from build123d import *

# Parameters (mm, degrees)
BOSS_EXTRUDE1_DEPTH     = 4.4
BOSS_EXTRUDE2_DEPTH     = 1.5
SKETCH3_W               = 42.21
SKETCH3_H               = 37.765
SKETCH3_W_2             = 5.0500889
SKETCH3_H_2             = 9.1998476
SKETCH3_W_3             = 9.1998476
SKETCH3_H_3             = 5.0500889
SKETCH3_W_4             = 12.70002032
SKETCH3_H_4             = 2.54
BOSS_EXTRUDE3_DEPTH     = 1.5
BOSS_EXTRUDE4_START     = -4.4
BOSS_EXTRUDE4_DEPTH     = 4.4
SKETCH4_R               = 0.85
CUT_EXTRUDE1_DEPTH      = 32.45281913
MIRROR2_START           = -4.4
MIRROR2_COPY_1_DEPTH    = 4.4
MIRROR2_COPY_2_SKETCH_R = 0.85
MIRROR2_COPY_2_DEPTH    = 32.45281913
FILLET1_R               = 0.5
SKETCH7_W               = 10
SKETCH7_H               = 1
CUT_EXTRUDE2_DEPTH      = 3
SKETCH8_W               = 1
SKETCH8_H               = 10
CUT_EXTRUDE3_DEPTH      = 3


with BuildPart() as part:
    # Sketch1 → Boss-Extrude1 (new body)
    with BuildSketch(Plane.XY):
        with BuildLine():
            Line((-19.431, 20.8825), (19.431, 20.8825))
            ThreePointArc((19.431, 20.8825), (22.028910314, 19.806410314), (23.105, 17.2085))
            Line((23.105, 17.2085), (23.105, -17.2085))
            ThreePointArc((23.105, -17.2085), (22.028910314, -19.806410314), (19.431, -20.8825))
            Line((19.431, -20.8825), (-19.431, -20.8825))
            ThreePointArc((-19.431, -20.8825), (-22.028910314, -19.806410314), (-23.105, -17.2085))
            Line((-23.105, -17.2085), (-23.105, 17.2085))
            ThreePointArc((-23.105, 17.2085), (-22.028910314, 19.806410314), (-19.431, 20.8825))
        make_face()
        with BuildLine():
            Line((-19.431, -18.8825), (19.431, -18.8825))
            ThreePointArc((19.431, -18.8825), (20.614696752, -18.392196752), (21.105, -17.2085))
            Line((21.105, -17.2085), (21.105, 17.2085))
            ThreePointArc((21.105, 17.2085), (20.614696752, 18.392196752), (19.431, 18.8825))
            Line((19.431, 18.8825), (-19.431, 18.8825))
            ThreePointArc((-19.431, 18.8825), (-20.614696752, 18.392196752), (-21.105, 17.2085))
            Line((-21.105, 17.2085), (-21.105, -17.2085))
            ThreePointArc((-21.105, -17.2085), (-20.614696752, -18.392196752), (-19.431, -18.8825))
        make_face(mode=Mode.SUBTRACT)
    extrude(amount=BOSS_EXTRUDE1_DEPTH)

    # Sketch2 → Boss-Extrude2 (add)
    with BuildSketch(Plane(origin=(0, 0, 0), x_dir=(-1, 0, 0), z_dir=(0, 0, -1))):
        with BuildLine():
            Line((21.105, 17.2085), (21.105, -17.2085))
            ThreePointArc((21.105, -17.2085), (20.614696752, -18.392196752), (19.431, -18.8825))
            Line((19.431, -18.8825), (-19.431, -18.8825))
            ThreePointArc((-19.431, -18.8825), (-20.614696752, -18.392196752), (-21.105, -17.2085))
            Line((-21.105, -17.2085), (-21.105, 17.2085))
            ThreePointArc((-21.105, 17.2085), (-20.614696752, 18.392196752), (-19.431, 18.8825))
            Line((-19.431, 18.8825), (19.431, 18.8825))
            ThreePointArc((19.431, 18.8825), (20.614696752, 18.392196752), (21.105, 17.2085))
        make_face()
    extrude(amount=-BOSS_EXTRUDE2_DEPTH)

    # Sketch3 → Boss-Extrude3 (add)
    with BuildSketch(Plane.XY.offset(1.5)):
        Rectangle(SKETCH3_W, SKETCH3_H)
        Polygon((-19.91503683, 15.787528575), (-4.21501143, 15.787528575), (-4.21501143, 2.627508255), (-11.83502667, 2.627508255), (-11.83502667, -2.452501905), (-19.91503683, -2.452501905), align=None, mode=Mode.SUBTRACT)
        Polygon((5.98500889, 15.707528575), (5.98500889, 12.207528575), (2.138501397, 12.207528575), (2.138501397, 2.707508255), (-2.528503937, 2.707508255), (-2.528503937, 15.707528575), align=None, mode=Mode.SUBTRACT)
        Polygon((16.498531877, 2.707508255), (16.498531877, 15.707528575), (11.831526543, 15.707528575), (11.831526543, 6.207508255), (7.98501905, 6.207508255), (7.98501905, 2.707508255), align=None, mode=Mode.SUBTRACT)
        with Locations((17.726060452, -6.667513335)):
            Rectangle(SKETCH3_W_2, SKETCH3_H_2, mode=Mode.SUBTRACT)
        with Locations((-13.33502667, -15.503556007)):
            Rectangle(SKETCH3_W_3, SKETCH3_H_3, mode=Mode.SUBTRACT)
        with Locations((14.60502921, -16.319532639)):
            Rectangle(SKETCH3_W_4, SKETCH3_H_4, mode=Mode.SUBTRACT)
    extrude(amount=BOSS_EXTRUDE3_DEPTH)

    # Sketch5 → Boss-Extrude4 (add)
    with BuildSketch(Plane.XY.offset(4.4).offset(BOSS_EXTRUDE4_START)):
        with BuildLine():
            Line((19.431, 20.8825), (21.605, 20.8825))
            ThreePointArc((21.605, 20.8825), (22.665660172, 20.443160172), (23.105, 19.3825))
            Line((23.105, 19.3825), (23.105, 17.2085))
            ThreePointArc((23.105, 17.2085), (22.028910314, 19.806410314), (19.431, 20.8825))
        make_face()
    boss_extrude4 = extrude(amount=BOSS_EXTRUDE4_DEPTH)

    # Sketch4 → Cut-Extrude1 (cut, through all)
    with BuildSketch(Plane.XY.offset(4.4)):
        with Locations((21.357158872, 19.134658872)):
            Circle(SKETCH4_R)
    cut_extrude1 = extrude(amount=-CUT_EXTRUDE1_DEPTH, mode=Mode.SUBTRACT)

    # Mirror1: Boss-Extrude4, Cut-Extrude1 across plane
    add(boss_extrude4.mirror(Plane(origin=(0, 0, 0), x_dir=(0, 0, 1), z_dir=(1, 0, 0))))
    add(cut_extrude1.mirror(Plane(origin=(0, 0, 0), x_dir=(0, 0, 1), z_dir=(1, 0, 0))), mode=Mode.SUBTRACT)

    # Mirror2: Boss-Extrude4, Cut-Extrude1 across plane
    add(boss_extrude4.mirror(Plane.ZX))
    add(cut_extrude1.mirror(Plane.ZX), mode=Mode.SUBTRACT)

    # Mirror2 copy 1 sketch → Mirror2 copy 1 (add)
    with BuildSketch(Plane(origin=(0, 0, 4.4), x_dir=(-1, 0, 0), z_dir=(0, 0, 1)).offset(MIRROR2_START)):
        with BuildLine():
            Line((19.431, 20.8825), (21.605, 20.8825))
            ThreePointArc((21.605, 20.8825), (22.665660172, 20.443160172), (23.105, 19.3825))
            Line((23.105, 19.3825), (23.105, 17.2085))
            ThreePointArc((23.105, 17.2085), (22.028910314, 19.806410314), (19.431, 20.8825))
        make_face()
    extrude(amount=MIRROR2_COPY_1_DEPTH)

    # Mirror2 copy 2 sketch → Mirror2 copy 2 (cut, through all)
    with BuildSketch(Plane(origin=(0, 0, 4.4), x_dir=(-1, 0, 0), z_dir=(0, 0, 1))):
        with Locations((21.357158872, 19.134658872)):
            Circle(MIRROR2_COPY_2_SKETCH_R)
    extrude(amount=-MIRROR2_COPY_2_DEPTH, mode=Mode.SUBTRACT)

    # Fillet1
    fillet1_edges = [part.edges().sort_by_distance(p)[0] for p in [
        (-23.105, 0, 0),
        (22.665660172, 20.443160172, 0),
        (-22.665660172, 20.443160172, 0),
        (-22.665660172, -20.443160172, 0),
        (22.665660172, -20.443160172, 0),
        (0, 20.8825, 0),
        (23.105, 0, 0),
        (0, -20.8825, 0),
    ]]
    fillet(fillet1_edges, radius=FILLET1_R)

    # Sketch7 → Cut-Extrude2 (cut)
    with BuildSketch(Plane.XZ.offset(20.8825)):
        with Locations((-13.33502667, 3.9)):
            Rectangle(SKETCH7_W, SKETCH7_H)
    extrude(amount=-CUT_EXTRUDE2_DEPTH, mode=Mode.SUBTRACT)

    # Sketch8 → Cut-Extrude3 (cut)
    with BuildSketch(Plane(origin=(23.105, 0, 0), x_dir=(0, 0, -1), z_dir=(1, 0, 0))):
        with Locations((-3.9, -6.667513335)):
            Rectangle(SKETCH8_W, SKETCH8_H)
    extrude(amount=-CUT_EXTRUDE3_DEPTH, mode=Mode.SUBTRACT)


solid = part.part
Can you work these out from the model? Positions are in its coordinate system, mm. A direction names the side the tool comes from. Give positions to 0.01 mm unless a question says otherwise; leave off trailing zeros. Loops run counter-clockwise (first coordinate to the right, second up) from the corner with the lowest first, then second, coordinate; pieces in that order, holes last. Notation, with made-up numbers: (-26, -39.5) -> (21, -39.5) arc R17 cw to (21, -20.5) -> close; hole circle Ø11 at (48.25, 45.5). An arc over 180 degrees is marked (long way). Return JSON: item names as keys, results as strings.
Q1. I want a section at C-C, the plane x = 10.5. List the corners of the cut face in (y, z) for me.
Checks:
{"outline": "(-20.88, 0.5) arc R0.5 ccw to (-20.38, 0) -> (20.38, 0) arc R0.5 ccw to (20.88, 0.5) -> (20.88, 4.4) -> (18.88, 4.4) -> (18.88, 3) -> (6.21, 3) -> (6.21, 1.5) -> (2.71, 1.5) -> (2.71, 3) -> (-15.05, 3) -> (-15.05, 1.5) -> (-17.59, 1.5) -> (-17.59, 3) -> (-18.88, 3) -> (-18.88, 4.4) -> (-20.88, 4.4) -> close"}
Q2. For pin 1 Ø1.4 at (x, y) = (-21.36, -19.13) entering from -Z; pin 2 Ø10 at (x, y) = (13.5, -2.5) entering from -Z; pin 3 Ø4.5 at (x, y) = (-11.5, 4.5) entering from +Z, each with a flat end and sliding along its axis, tell me the tip position at first contact or that it passes through.
Checks:
{"pin 1": "passes through", "pin 2": "stops at z = 0", "pin 3": "stops at z = 3"}
Q3. I want a section at A-A, the plane x = 0.5. List the corners of the cut face in (y, z) for me, then the cut area to 3 significant figures.
Checks:
{"outline": "(-20.88, 0.5) arc R0.5 ccw to (-20.38, 0) -> (20.38, 0) arc R0.5 ccw to (20.88, 0.5) -> (20.88, 4.4) -> (18.88, 4.4) -> (18.88, 3) -> (15.71, 3) -> (15.71, 1.5) -> (2.71, 1.5) -> (2.71, 3) -> (-18.88, 3) -> (-18.88, 4.4) -> (-20.88, 4.4) -> close", "area": "111 mm2"}
Q4. We'd pull the mould along X, two halves only. Please class faces 4 (the face through (20.508, 19.172, 2.231)), 5 (the face through (-23.105, 0, 2)), 6 (the face through (0, 20.882, 2)): released by +X, released by -X, zero draft, split by the parting line, or undercut.
Checks:
{"face 4": "undercut", "face 5": "released by -X", "face 6": "zero draft"}
Q5. On a 3-axis mill with a long thin cutter (end or side, diameter ignored), from which of +Z, -Z, +X, -X, +Y, -Y can I reach the whole of each face in a straight line? I mean faces 1 (the face through (-11.835, 0, 2)), 2 (the face through (-13, -20, 3.4)), 3 (the face through (22.654, -20.455, 2.423)). Say none if no direction works.
Checks:
{"face 1": "+Z", "face 2": "+Z, -Y", "face 3": "+Z, -Z, +X, -Y"}
Q6. I need wall thicknesses on probe 1 along X at (y, z) = (15, 1.55) (1 decimal); probe 2 along Y at (x, z) = (-13.5, 2.2); probe 3 along X at (y, z) = (-14.5, 2.3) (3 decimals). Which ranges of each line are inside material? Lowest first, please.
Checks:
{"probe 1": "x = -23.1 to -19.9, -4.2 to -2.5, 6 to 11.8, 16.5 to 23.1", "probe 2": "y = -20.88 to -18.03, -12.98 to -2.45, 15.79 to 20.88", "probe 3": "x = -23.105 to -17.935, -8.735 to 23.105"}
Q7. I want a section at D-D, the plane y = -16. List the corners of the cut face in (x, z) for me (3 decimals).
Checks:
{"outline": "(-23.105, 0.5) arc R0.5 ccw to (-22.605, 0) -> (22.605, 0) arc R0.5 ccw to (23.105, 0.5) -> (23.105, 4.4) -> (21.105, 4.4) -> (21.105, 3) -> (20.955, 3) -> (20.955, 1.5) -> (8.255, 1.5) -> (8.255, 3) -> (-8.735, 3) -> (-8.735, 1.5) -> (-17.935, 1.5) -> (-17.935, 3) -> (-21.105, 3) -> (-21.105, 4.4) -> (-23.105, 4.4) -> close"}
Q8. I want a section at B-B, the plane y = -6. List the corners of the cut face in (x, z) for me (3 decimals).
Checks:
{"outline": "(-23.105, 0.5) arc R0.5 ccw to (-22.605, 0) -> (22.605, 0) arc R0.5 ccw to (23.105, 0.5) -> (23.105, 3.4) -> (21.105, 3.4) -> (21.105, 3) -> (20.251, 3) -> (20.251, 1.5) -> (15.201, 1.5) -> (15.201, 3) -> (-21.105, 3) -> (-21.105, 4.4) -> (-23.105, 4.4) -> close"}
